Here's how the part is built. I have some questions about the finished solid (model axes, mm). Give positions to 0.01 mm unless a question says otherwise; leave off trailing zeros. Answer in a Markdown table with one row per item. Add a question column.
Item 1: If we section it at A-A (y = 1.1): Give the number of separate pieces and of enclosed holes in the cut face, then the cut area to 3 significant figures.
Item 2: For P1, Ø2.5, axis at x = 75.65, z = 222.66, coming from the +Y side; P2, Ø1, axis at y = 0.5, z = -19.5, coming from the -X side, each with a flat end and sliding along its axis, tell me the tip position at first contact or that it passes through.
Item 3: If I drill on line 1 (Z direction, x = 12, y = 2.45); line 2 (Z direction, x = 200.5, y = 2.95); line 3 (X direction, y = 2.15, z = 73), over which ranges is the centre line in solid material (lowest first)?
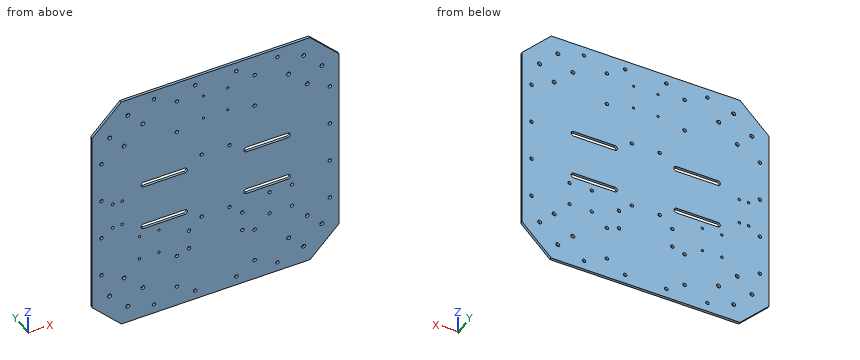
```python
from build123d import *

# Parameters (mm, degrees)
BOSS_EXTRUDE1_DEPTH = 3.175
SKETCH2_R           = 2.4638
CUT_EXTRUDE1_DEPTH  = 6.35
SKETCH3_R           = 2.159
CUT_EXTRUDE2_DEPTH  = 6.35
SKETCH4_R           = 2.2225
CUT_EXTRUDE3_DEPTH  = 351.937720963
SKETCH5_R           = 1.651
CUT_EXTRUDE4_DEPTH  = 351.937720963
SKETCH6_R           = 2.032
SKETCH6_R_2         = 2.159
SKETCH6_R_3         = 1.397
SKETCH6_R_4         = 1.5499969
CUT_EXTRUDE5_DEPTH  = 351.937720963
SKETCH7_R           = 2.159
CUT_EXTRUDE6_DEPTH  = 351.937720963


with BuildPart() as part:
    # Sketch1 → Boss-Extrude1 (new body)
    with BuildSketch(Plane(origin=(0, 0, 0), x_dir=(1, 0, 0), z_dir=(0, 1, 0))):
        Polygon((-25.845025354, 51.656360067), (-61.766049839, 15.735335583), (-61.766049839, -217.222615449), (-25.845025354, -253.143639933), (207.112925677, -253.143639933), (243.033950161, -217.222615449), (243.033950161, 15.735335583), (207.112925677, 51.656360067), align=None)
        with BuildLine():
            ThreePointArc((52.533950161, -126.143639933), (55.708950161, -129.318639933), (52.533950161, -132.493639933))
            Line((52.533950161, -132.493639933), (1.733950161, -132.493639933))
            ThreePointArc((1.733950161, -132.493639933), (-1.441049839, -129.318639933), (1.733950161, -126.143639933))
            Line((1.733950161, -126.143639933), (52.533950161, -126.143639933))
        make_face(mode=Mode.SUBTRACT)
        with BuildLine():
            Line((179.533950161, -132.493639933), (128.733950161, -132.493639933))
            ThreePointArc((128.733950161, -132.493639933), (125.558950161, -129.318639933), (128.733950161, -126.143639933))
            Line((128.733950161, -126.143639933), (179.533950161, -126.143639933))
            ThreePointArc((179.533950161, -126.143639933), (182.708950161, -129.318639933), (179.533950161, -132.493639933))
        make_face(mode=Mode.SUBTRACT)
        with BuildLine():
            Line((1.733950161, -68.993639933), (52.533950161, -68.993639933))
            ThreePointArc((52.533950161, -68.993639933), (55.708950161, -72.168639933), (52.533950161, -75.343639933))
            Line((52.533950161, -75.343639933), (1.733950161, -75.343639933))
            ThreePointArc((1.733950161, -75.343639933), (-1.441049839, -72.168639933), (1.733950161, -68.993639933))
        make_face(mode=Mode.SUBTRACT)
        with BuildLine():
            ThreePointArc((128.733950161, -75.343639933), (125.558950161, -72.168639933), (128.733950161, -68.993639933))
            Line((128.733950161, -68.993639933), (179.533950161, -68.993639933))
            ThreePointArc((179.533950161, -68.993639933), (182.708950161, -72.168639933), (179.533950161, -75.343639933))
            Line((179.533950161, -75.343639933), (128.733950161, -75.343639933))
        make_face(mode=Mode.SUBTRACT)
    extrude(amount=BOSS_EXTRUDE1_DEPTH)

    # Sketch2 → Cut-Extrude1 (cut)
    with BuildSketch(Plane(origin=(0, 3.175, 0), x_dir=(1, 0, 0), z_dir=(0, 1, 0))):
        with Locations(Location((-17.872380726, 30.213331256, 0), (0, 0, 270))):
            Circle(SKETCH2_R)
        with Locations(Location((0.640891541, 11.70005899, 0), (0, 0, 270))):
            Circle(SKETCH2_R)
        with Locations(Location((-22.362508786, -10.197821288, 0), (0, 0, 270))):
            Circle(SKETCH2_R)
        with Locations(Location((-40.323021028, 7.762690954, 0), (0, 0, 270))):
            Circle(SKETCH2_R)
        with Locations(Location((203.630409109, -10.197821288, 0), (0, 0, 270))):
            Circle(SKETCH2_R)
        with Locations(Location((221.590921351, 7.762690954, 0), (0, 0, 270))):
            Circle(SKETCH2_R)
        with Locations(Location((180.627008782, 11.70005899, 0), (0, 0, 270))):
            Circle(SKETCH2_R)
        with Locations(Location((199.140281048, 30.213331256, 0), (0, 0, 270))):
            Circle(SKETCH2_R)
        with Locations(Location((-22.362508786, -191.289458578, 0), (0, 0, 270))):
            Circle(SKETCH2_R)
        with Locations(Location((-40.323021028, -209.24997082, 0), (0, 0, 270))):
            Circle(SKETCH2_R)
        with Locations(Location((-17.872380726, -231.700611123, 0), (0, 0, 270))):
            Circle(SKETCH2_R)
        with Locations(Location((0.640891541, -213.187338857, 0), (0, 0, 270))):
            Circle(SKETCH2_R)
        with Locations(Location((221.590921351, -209.24997082, 0), (0, 0, 270))):
            Circle(SKETCH2_R)
        with Locations(Location((199.140281048, -231.700611123, 0), (0, 0, 270))):
            Circle(SKETCH2_R)
        with Locations(Location((180.627008782, -213.187338857, 0), (0, 0, 270))):
            Circle(SKETCH2_R)
        with Locations(Location((203.630409109, -191.289458578, 0), (0, 0, 270))):
            Circle(SKETCH2_R)
    extrude(amount=-CUT_EXTRUDE1_DEPTH, mode=Mode.SUBTRACT)

    # Sketch3 → Cut-Extrude2 (cut)
    with BuildSketch(Plane(origin=(0, 3.175, 0), x_dir=(1, 0, 0), z_dir=(0, 1, 0))):
        with Locations(Location((73.361950161, -58.198639933, 0), (0, 0, 270))):
            Circle(SKETCH3_R)
        with Locations(Location((107.651950161, -58.198639933, 0), (0, 0, 270))):
            Circle(SKETCH3_R)
        with Locations(Location((73.361950161, -143.288639933, 0), (0, 0, 270))):
            Circle(SKETCH3_R)
        with Locations(Location((107.651950161, -143.288639933, 0), (0, 0, 270))):
            Circle(SKETCH3_R)
    extrude(amount=-CUT_EXTRUDE2_DEPTH, mode=Mode.SUBTRACT)

    # Sketch4 → Cut-Extrude3 (cut, through all)
    with BuildSketch(Plane(origin=(0, 3.175, 0), x_dir=(1, 0, 0), z_dir=(0, 1, 0))):
        with Locations(Location((42.754950161, 26.256360067, 0), (0, 0, 270))):
            Circle(SKETCH4_R)
        with Locations(Location((138.512950161, 26.256360067, 0), (0, 0, 270))):
            Circle(SKETCH4_R)
        with Locations(Location((42.754950161, -15.653639933, 0), (0, 0, 270))):
            Circle(SKETCH4_R)
        with Locations(Location((138.512950161, -15.653639933, 0), (0, 0, 270))):
            Circle(SKETCH4_R)
        with Locations(Location((138.512950161, -185.833639933, 0), (0, 0, 90))):
            Circle(SKETCH4_R)
        with Locations(Location((42.754950161, -185.833639933, 0), (0, 0, 90))):
            Circle(SKETCH4_R)
        with Locations(Location((138.512950161, -227.743639933, 0), (0, 0, 90))):
            Circle(SKETCH4_R)
        with Locations(Location((42.754950161, -227.743639933, 0), (0, 0, 90))):
            Circle(SKETCH4_R)
    extrude(amount=-CUT_EXTRUDE3_DEPTH, mode=Mode.SUBTRACT)

    # Sketch5 → Cut-Extrude4 (cut, through all)
    with BuildSketch(Plane(origin=(0, 3.175, 0), x_dir=(1, 0, 0), z_dir=(0, 1, 0))):
        with Locations(Location((-36.366049839, -84.741639933, 0), (0, 0, 270))):
            Circle(SKETCH5_R)
        with Locations(Location((-24.936049839, -84.741639933, 0), (0, 0, 270))):
            Circle(SKETCH5_R)
        with Locations(Location((-24.936049839, -116.745639933, 0), (0, 0, 90))):
            Circle(SKETCH5_R)
        with Locations(Location((-36.366049839, -116.745639933, 0), (0, 0, 90))):
            Circle(SKETCH5_R)
    extrude(amount=-CUT_EXTRUDE4_DEPTH, mode=Mode.SUBTRACT)

    # Sketch6 → Cut-Extrude5 (cut, through all)
    with BuildSketch(Plane(origin=(0, 3.175, 0), x_dir=(1, 0, 0), z_dir=(0, 1, 0))):
        with Locations(Location((157.181950161, -30.893639933, 0), (0, 0, 270))):
            Circle(SKETCH6_R)
        with Locations(Location((157.181950161, -59.849639933, 0), (0, 0, 270))):
            Circle(SKETCH6_R)
        with Locations(Location((184.613950161, -59.849639933, 0), (0, 0, 270))):
            Circle(SKETCH6_R)
        with Locations(Location((184.613950161, -30.893639933, 0), (0, 0, 270))):
            Circle(SKETCH6_R)
        with Locations(Location((57.613950161, -20.733639933, 0), (0, 0, 270))):
            Circle(SKETCH6_R_2)
        with Locations(Location((57.613950161, -44.863639933, 0), (0, 0, 270))):
            Circle(SKETCH6_R_2)
        with Locations(Location((123.653950161, -44.863639933, 0), (0, 0, 90))):
            Circle(SKETCH6_R_2)
        with Locations(Location((123.653950161, -20.733639933, 0), (0, 0, 90))):
            Circle(SKETCH6_R_2)
        with Locations(Location((75.647950161, -192.691639933, 0), (0, 0, 270))):
            Circle(SKETCH6_R_3)
        with Locations(Location((75.647950161, -222.663639933, 0), (0, 0, 270))):
            Circle(SKETCH6_R_3)
        with Locations(Location((105.619950161, -222.663639933, 0), (0, 0, 90))):
            Circle(SKETCH6_R_3)
        with Locations(Location((105.619950161, -192.691639933, 0), (0, 0, 90))):
            Circle(SKETCH6_R_3)
        with Locations(Location((-3.388950787, -29.369639933, 0), (0, 0, 270))):
            Circle(SKETCH6_R_4)
        with Locations(Location((-3.346049839, -59.769599662, 0), (0, 0, 270))):
            Circle(SKETCH6_R_4)
        with Locations(Location((20.611052013, -29.369639933, 0), (0, 0, 270))):
            Circle(SKETCH6_R_4)
        with Locations(Location((20.611052013, -59.769599662, 0), (0, 0, 270))):
            Circle(SKETCH6_R_4)
    extrude(amount=-CUT_EXTRUDE5_DEPTH, mode=Mode.SUBTRACT)

    # Sketch7 → Cut-Extrude6 (cut, through all)
    with BuildSketch(Plane(origin=(0, 3.175, 0), x_dir=(1, 0, 0), z_dir=(0, 1, 0))):
        with Locations(Location((65.233950161, 40.226360067, 0), (0, 0, 270))):
            Circle(SKETCH7_R)
        with Locations(Location((14.433950161, 40.226360067, 0), (0, 0, 270))):
            Circle(SKETCH7_R)
        with Locations(Location((-50.336049839, -75.343639933, 0), (0, 0, 270))):
            Circle(SKETCH7_R)
        with Locations(Location((-50.336049839, -24.543639933, 0), (0, 0, 270))):
            Circle(SKETCH7_R)
        with Locations(Location((231.603950161, -24.543639933, 0), (0, 0, 90))):
            Circle(SKETCH7_R)
        with Locations(Location((231.603950161, -75.343639933, 0), (0, 0, 90))):
            Circle(SKETCH7_R)
        with Locations(Location((166.833950161, 40.226360067, 0), (0, 0, 90))):
            Circle(SKETCH7_R)
        with Locations(Location((116.033950161, 40.226360067, 0), (0, 0, 90))):
            Circle(SKETCH7_R)
        with Locations(Location((116.033950161, -241.713639933, 0), (0, 0, 270))):
            Circle(SKETCH7_R)
        with Locations(Location((166.833950161, -241.713639933, 0), (0, 0, 270))):
            Circle(SKETCH7_R)
        with Locations(Location((231.603950161, -126.143639933, 0), (0, 0, 270))):
            Circle(SKETCH7_R)
        with Locations(Location((231.603950161, -176.943639933, 0), (0, 0, 270))):
            Circle(SKETCH7_R)
        with Locations(Location((-50.336049839, -176.943639933, 0), (0, 0, 90))):
            Circle(SKETCH7_R)
        with Locations(Location((-50.336049839, -126.143639933, 0), (0, 0, 90))):
            Circle(SKETCH7_R)
        with Locations(Location((14.433950161, -241.713639933, 0), (0, 0, 90))):
            Circle(SKETCH7_R)
        with Locations(Location((65.233950161, -241.713639933, 0), (0, 0, 90))):
            Circle(SKETCH7_R)
    extrude(amount=-CUT_EXTRUDE6_DEPTH, mode=Mode.SUBTRACT)


solid = part.part
```
Recorded:
| question | item | result |
|---|---|---|
| 1 | separate pieces | 1 |
| 1 | enclosed holes | 68 |
| 1 | area | 88,000 mm^2 |
| 2 | P1 | passes through |
| 2 | P2 | stops at x = -58.5 |
| 3 | line 1 | z = -51.66 to 68.99, 75.34 to 126.14, 132.49 to 253.14 |
| 3 | line 2 | z = -51.66 to -32.27, -28.16 to 229.65, 233.76 to 253.14 |
| 3 | line 3 | x = -61.77 to -1.33, 55.6 to 125.67, 182.6 to 243.03 |
